```python
from build123d import *

# Parameters (mm, degrees)
SKETCH_R     = 3.9
SKETCH_R_2   = 2.9
PAD_DEPTH    = 10
SKETCH001_W  = 6.4
SKETCH001_H  = 7.8
POCKET_DEPTH = 5.001
PAD001_DEPTH = 1
FILLET_R     = 0.2
FILLET001_R  = 0.2


with BuildPart() as part:
    # Sketch → Pad (new body)
    with BuildSketch(Plane.XY):
        Circle(SKETCH_R)
        Circle(SKETCH_R_2, mode=Mode.SUBTRACT)
    extrude(amount=PAD_DEPTH)

    # Sketch001 → Pocket (cut, through all)
    with BuildSketch(Plane.XY.offset(5)):
        with Locations((0.7, 0)):
            Rectangle(SKETCH001_W, SKETCH001_H)
    extrude(amount=POCKET_DEPTH, mode=Mode.SUBTRACT)

    # Sketch002 → Pad001 (join)
    with BuildSketch(Plane.XY.offset(9)):
        with BuildLine():
            ThreePointArc((-4.301793, 2.346184), (-4.9, 0), (-4.301793, -2.346184))
            Line((-4.301793, -2.346184), (-3.115352, -2.346184))
            ThreePointArc((-3.115352, 2.346184), (-3.9, 0), (-3.115352, -2.346184))
            Line((-4.301793, 2.346184), (-3.115352, 2.346184))
        make_face()
    extrude(amount=PAD001_DEPTH)

    # Fillet
    fillet_edges = [part.edges().sort_by_distance(p)[0] for p in [
        (-2.5, -2.993326, 7.5),
        (-2.5, 2.993326, 7.5),
    ]]
    fillet(fillet_edges, radius=FILLET_R)

    # Fillet001
    fillet001_edges = [part.edges().sort_by_distance(p)[0] for p in [
        (-4.301793, 2.346184, 9.5),
        (-4.301793, -2.346184, 9.5),
        (-4.9, 0, 9),
        (-4.9, 0, 10),
    ]]
    fillet(fillet001_edges, radius=FILLET001_R)


solid = part.part
```
Design review of the part built by this model. Coordinates are the model's own, in mm. A direction names the side the tool comes from. Round coordinates to 2 decimals unless told otherwise and drop trailing zeros. Write each loop counter-clockwise with the first axis right and the second up, starting at its lowest first coordinate (ties: lowest second). Pieces come first, ordered by that corner, then holes.
Item 1: Clearance check with flat-ended pins moving along their axes: pin 1 Ø4 at (y, z) = (-1.5, 2) entering from +X; pin 2 Ø3.5 at (x, y) = (0, 0) entering from +Z; pin 3 Ø0.5 at (y, z) = (2, 7.5) entering from +X; pin 4 Ø0.5 at (x, z) = (-3.5, 9.5) entering from +Y. State where each tip first meets the part, or that it passes through.
Item 2: We need section C-C on z = 4. Write out the cut boundary in (x, y), and give its area (3 significant figures).
Item 3: For faces 1 (the flat face through (-2.5, -2, 7)), 2 (the flat face through (-1, 3, 0)), 3 (the flat face through (-3.7, 2.346, 9.5)), 4 (the flat face through (-3.7, -2.346, 9.5)), list the 3-axis set-ups (+Z, -Z, +X, -X, +Y, -Y) from which the entire face can be reached by the end or side of a thin tool; tool diameter is ignored.
Item 4: We need section B-B on y = 0. Write out the cut boundary in (x, z), and give its area (3 significant figures).
Item 5: For probe 1 along Y at (x, z) = (0, 4); probe 2 along Z at (x, y) = (-4, -1.25); probe 3 along Z at (x, y) = (-1.5, -3.5), list the stretches that pass through material, from the lowest coordinate up.
Item 6: We need section D-D on x = 2.25. Write out the cut boundary in (y, z), and give its area (3 significant figures).
Item 7: The part is to be moulded in two halves that separate along X. For faces 5 (the cylindrical face through (-2.9, 0.1, 2.7)), 6 (the cylindrical face through (-3.896, 0.171, 3.819)), 7 (the flat face through (-4, 0, 10)), say which applies: +X half, -X half, draft (parallel to the pull), parting line (faces both ways), or undercut.
Item 8: We need section A-A on x = 0. Write out the cut boundary in (y, z), and give its area (3 significant figures).
Returned:
1. pin 1: stops at x = 3.9
1. pin 2: passes through
1. pin 3: stops at x = -2.5
1. pin 4: stops at y = 2.35
2. outline: circle Ø7.8 at (0, 0); hole circle Ø5.8 at (0, 0)
2. area: 21.4 mm2
3. face 1: +Z, +X, +Y, -Y
3. face 2: -Z, +X, -X, +Y, -Y
3. face 3: +Z, -Z, -X, +Y
3. face 4: +Z, -Z, -X, -Y
4. outline: (-4.9, 9.2) arc R0.2 ccw to (-4.7, 9) - (-3.9, 9) - (-3.9, 0) - (-2.9, 0) - (-2.9, 10) - (-4.7, 10) arc R0.2 ccw to (-4.9, 9.8) - close; (2.9, 0) - (3.9, 0) - (3.9, 5) - (2.9, 5) - close
4. area: 16.0 mm2
5. probe 1: y = -3.9 to -2.9, 2.9 to 3.9
5. probe 2: z = 9 to 10
5. probe 3: z = 0 to 5
6. outline: (-3.19, 0) - (-1.83, 0) - (-1.83, 5) - (-3.19, 5) - close; (1.83, 0) - (3.19, 0) - (3.19, 5) - (1.83, 5) - close
6. area: 13.6 mm2
7. face 5: undercut
7. face 6: parting line
7. face 7: draft
8. outline: (-3.9, 0) - (-2.9, 0) - (-2.9, 5) - (-3.9, 5) - close; (2.9, 0) - (3.9, 0) - (3.9, 5) - (2.9, 5) - close
8. area: 10.0 mm2
